CAD build for the part. Positions are in the model's coordinates, mm. A direction names the side the tool comes from. Coordinates: 2 decimals unless noted, no trailing zeros. Write each loop counter-clockwise with the first axis right and the second up, starting at its lowest first coordinate (ties: lowest second). Pieces come first, ordered by that corner, then holes.
```python
from build123d import *

# Parameters (mm, degrees)
F0_W      = 152.4
F0_H      = 38.1
F1_DEPTH  = 6.35
F2_R      = 2.0447
F3_DEPTH  = 76.2
F4_DEPTH  = 76.2
F5_R      = 2.7305
F6_DEPTH  = 1.016
F8_DEPTH  = 7.62
F9_R      = 3.5941
F10_DEPTH = 1.905
F11_R     = 4.7625
F12_DEPTH = 0.635
F13_R     = 1.524
F14_DEPTH = 1.00076
F15_W     = 25.4
F15_H     = 38.1
F16_DEPTH = 7.62
F18_DEPTH = 1.27
F19_R     = 3.2131
F20_DEPTH = 0.508
F22_DEPTH = 0.762
F23_R     = 2.032
F24_DEPTH = 8.382
F25_R     = 3.048
F26_DEPTH = 0.3556
F27_R     = 2.9718
F28_DEPTH = 0.6604
F29_R     = 2.6162
F30_DEPTH = 1.1176
F31_R     = 2.9845
F32_DEPTH = 13.7922
F33_R     = 3.175
F34_DEPTH = 6.35
F36_DEPTH = 2.7305
F37_W     = 20.3219614923
F37_H     = 25.3980793059
F38_DEPTH = 25.4


with BuildPart() as f1:
    # F0 (on Top) → F1 (new body)
    with BuildSketch(Plane.XY):
        Rectangle(F0_W, F0_H)
    extrude(amount=F1_DEPTH)

    # F2 (on face) → F3 (join)
    with BuildSketch(Plane.YZ.offset(76.2)):
        with Locations((0, 6.35)):
            Circle(F2_R)
    extrude(amount=-F3_DEPTH)

    # F2 (on face) → F4 (cut)
    with BuildSketch(Plane.YZ.offset(76.2)):
        with Locations((0, 6.35)):
            Circle(F2_R)
    extrude(amount=-F4_DEPTH, mode=Mode.SUBTRACT)

    # F5 (on face) → F6 (cut)
    with BuildSketch(Plane.YZ):
        with Locations((0, 6.35)):
            Circle(F5_R)
    extrude(amount=-F6_DEPTH, mode=Mode.SUBTRACT)

    # F7 (on face) → F8 (cut)
    with BuildSketch(Plane.YZ.offset(-1.016)):
        with BuildLine():
            ThreePointArc((-2.4118311998, 6.35), (-0.1004311998, 4.0386), (2.2109688002, 6.35))
            Line((2.2109688002, 6.35), (-2.4118311998, 6.35))
        make_face()
    extrude(amount=-F8_DEPTH, mode=Mode.SUBTRACT)

    # F9 (on face) → F10 (cut)
    with BuildSketch(Plane.YZ.offset(-8.636)):
        with Locations((-0.1004311998, 6.35)):
            Circle(F9_R)
    extrude(amount=F10_DEPTH, mode=Mode.SUBTRACT)

    # F11 (on face) → F12 (cut)
    with BuildSketch(Plane.YZ.offset(-8.636)):
        with Locations((0, 6.35)):
            Circle(F11_R)
        with BuildLine():
            ThreePointArc((3.4936688002, 6.35), (-0.1004311998, 2.7559), (-3.6945311998, 6.35))
            Line((-3.6945311998, 6.35), (3.4936688002, 6.35))
        make_face(mode=Mode.SUBTRACT)
    extrude(amount=F12_DEPTH, mode=Mode.SUBTRACT)

    # F13 (on face) → F14 (cut)
    with BuildSketch(Plane.YZ.offset(-8.636)):
        with Locations((0, 6.35)):
            Circle(F13_R)
    extrude(amount=-F14_DEPTH, mode=Mode.SUBTRACT)

    # F15 (on face) → F16 (cut)
    with BuildSketch(Plane.YZ.offset(-9.63676)):
        with Locations((0, 6.35)):
            Rectangle(F15_W, F15_H)
    extrude(amount=-F16_DEPTH, mode=Mode.SUBTRACT)

    # F17 (on face) → F18 (cut)
    with BuildSketch(Plane.YZ.offset(-17.25676)):
        with BuildLine():
            ThreePointArc((-1.524, 6.35), (0, 4.826), (1.524, 6.35))
            Line((1.524, 6.35), (-1.524, 6.35))
        make_face()
        with BuildLine():
            Line((-1.524, 6.35), (1.524, 6.35))
            ThreePointArc((1.524, 6.35), (0, 7.874), (-1.524, 6.35))
        make_face()
    extrude(amount=-F18_DEPTH, mode=Mode.SUBTRACT)

    # F19 (on face) → F20 (cut)
    with BuildSketch(Plane.YZ.offset(-18.52676)):
        with Locations((0, 6.35)):
            Circle(F19_R)
        with BuildLine():
            ThreePointArc((1.524, 6.35), (0, 4.826), (-1.524, 6.35))
            Line((-1.524, 6.35), (1.524, 6.35))
        make_face(mode=Mode.SUBTRACT)
    extrude(amount=F20_DEPTH, mode=Mode.SUBTRACT)

    # F21 (on face) → F22 (cut)
    with BuildSketch(Plane.YZ.offset(-18.52676)):
        with BuildLine():
            ThreePointArc((-2.9337, 6.35), (0, 3.4163), (2.9337, 6.35))
            Line((2.9337, 6.35), (-2.9337, 6.35))
        make_face()
        with BuildLine():
            Line((-2.9337, 6.35), (2.9337, 6.35))
            ThreePointArc((2.9337, 6.35), (0, 9.2837), (-2.9337, 6.35))
        make_face()
    extrude(amount=-F22_DEPTH, mode=Mode.SUBTRACT)

    # F23 (on face) → F24 (cut)
    with BuildSketch(Plane.YZ.offset(-19.28876)):
        with Locations((0, 6.35)):
            Circle(F23_R)
    extrude(amount=-F24_DEPTH, mode=Mode.SUBTRACT)

    # F25 (on face) → F26 (cut)
    with BuildSketch(Plane.YZ.offset(-27.67076)):
        with Locations((0, 6.35)):
            Circle(F25_R)
    extrude(amount=-F26_DEPTH, mode=Mode.SUBTRACT)

    # F27 (on face) → F28 (cut)
    with BuildSketch(Plane.YZ.offset(-28.02636)):
        with Locations((0, 6.35)):
            Circle(F27_R)
    extrude(amount=-F28_DEPTH, mode=Mode.SUBTRACT)

    # F29 (on face) → F30 (cut)
    with BuildSketch(Plane.YZ.offset(-28.68676)):
        with Locations((0, 6.35)):
            Circle(F29_R)
    extrude(amount=-F30_DEPTH, mode=Mode.SUBTRACT)

    # F31 (on face) → F32 (cut)
    with BuildSketch(Plane.YZ.offset(-29.80436)):
        with Locations((0, 6.35)):
            Circle(F31_R)
    extrude(amount=-F32_DEPTH, mode=Mode.SUBTRACT)

    # F33 (on face) → F34 (join)
    with BuildSketch(Plane.XY.offset(6.35)):
        with Locations((-69.215, 12.065)):
            Circle(F33_R)
        with Locations((69.215, 12.065)):
            Circle(F33_R)
    extrude(amount=F34_DEPTH)

    # F35 (on face) → F36 (cut)
    with BuildSketch(Plane.XY.offset(6.35)):
        Polygon((1.016, 2.0447), (0, 2.7305), (0, -2.7305), (1.016, -2.0447), align=None)
    extrude(amount=-F36_DEPTH, mode=Mode.SUBTRACT)

    # F37 (on face) → F38 (cut)
    with BuildSketch(Plane.XY.offset(6.35)):
        with Locations((-13.3582856506, 0)):
            Rectangle(F37_W, F37_H)
    extrude(amount=-F38_DEPTH, mode=Mode.SUBTRACT)


solid = f1.part
```
Item 1: Saw through at C-C, the plane z = 7.75. Write the cut outline in (x, y) (3 decimals), and give its area (3 significant figures).
Item 2: Saw through at D-D, the plane x = -58.5. Write the cut outline in (y, z), and give its area (3 significant figures).
Item 3: Saw through at B-B, the plane x = 54. Write the cut outline in (y, z).
Item 4: Wall check: line 1 along X through (y, z) = (1, 4); line 2 along X through (y, z) = (-5, 3.5); line 3 along Y through (x, z) = (-22, 1.5). Give the ranges that are in metal, low to high.
Item 5: Flat gauge pins, fed straight in: pin 1 Ø2 at (x, y) = (32.5, -9) entering from +Z; pin 2 Ø4 at (x, z) = (5, 10) entering from +Y. Where does each tip first touch, or does it go through?
Item 6: Saw through at A-A, the plane y = 6. Write the cut outline in (x, z).
Item 7: Which spindle directions (+Z, -Z, +X, -X, +Y, -Y) get a long thin tool onto all of the face, cutting with end or side? Do faces 1 (the flat face through (-23.519, 0, 3)), 2 (the flat face through (-29.804, -0.5, 3.6)), 3 (the cylindrical face through (39.134, -0.045, 4.306)). Say none if no direction does.
Item 8: Two-plate mould, pull along Y, no slides. Class faces 4 (the flat face through (-1, 19.05, 3)), 5 (the flat face through (-6, 12.699, 3)), 6 (the cylindrical face through (72.243, 13.019, 9.481)): +Y half, -Y half, draft (parallel to the pull), parting line (faces both ways), or undercut.
Working result:
1. outline: circle Ø6.35 at (-69.215, 12.065); circle Ø6.35 at (69.215, 12.065)
1. area: 63.3 mm2
2. outline: (-19.05, 0) - (19.05, 0) - (19.05, 6.35) - (-19.05, 6.35) - close
2. area: 242 mm2
3. outline: (-19.05, 0) - (19.05, 0) - (19.05, 6.35) - (2.04, 6.35) arc R2.04 cw to (-2.04, 6.35) - (-19.05, 6.35) - close
4. line 1: x = -76.2 to -43.6, -27.67 to -23.52, -3.2 to -1.02, 1.02 to 76.2
4. line 2: x = -76.2 to -23.52, -3.2 to 76.2
4. line 3: y = -19.05 to -12.7, 12.7 to 19.05
5. pin 1: stops at z = 6.35
5. pin 2: passes through
6. outline: (-76.2, 0) - (-23.52, 0) - (-23.52, 6.35) - (-76.2, 6.35) - close; (-3.2, 0) - (76.2, 0) - (76.2, 6.35) - (-3.2, 6.35) - close
7. face 1: +Z, -Z
7. face 2: +Z
7. face 3: +Z, +X
8. face 4: +Y half
8. face 5: undercut
8. face 6: parting line
